The listing builds one solid part. Answer for the finished solid, in the listing's coordinates (mm). A direction names the side the tool comes from. Give positions to 0.01 mm unless a question says otherwise; leave off trailing zeros.
```python
from build123d import *

# Parameters (mm, degrees)
SKETCH1_W               = 60
SKETCH1_H               = 54.7
BOSS_EXTRUDE1_DEPTH     = 6.35
SKETCH2_W               = 15
SKETCH2_H               = 6
BOSS_EXTRUDE2_DEPTH     = 6.35
SKETCH3_R               = 1
CUT_EXTRUDE1_DEPTH      = 7.35
MIRROR2_COPY_1_SKETCH_W = 15
MIRROR2_COPY_1_SKETCH_H = 6
MIRROR2_COPY_1_DEPTH    = 6.35
MIRROR2_COPY_2_SKETCH_R = 1
MIRROR2_COPY_2_DEPTH    = 7.35
FILLET1_R               = 1
FILLET2_R               = 2


with BuildPart() as part:
    # Sketch1 → Boss-Extrude1 (new body)
    with BuildSketch(Plane.XY):
        Rectangle(SKETCH1_W, SKETCH1_H)
    extrude(amount=BOSS_EXTRUDE1_DEPTH)

    # Sketch2 → Boss-Extrude2 (add)
    with BuildSketch(Plane.XY.offset(6.35)):
        with Locations((-17.5, 30.35)):
            Rectangle(SKETCH2_W, SKETCH2_H)
    boss_extrude2 = extrude(amount=-BOSS_EXTRUDE2_DEPTH)

    # Sketch3 → Cut-Extrude1 (cut, through all)
    with BuildSketch(Plane.XY.offset(6.35)):
        with Locations((-25, 27.35)):
            Circle(SKETCH3_R)
        with Locations((-10, 27.35)):
            Circle(SKETCH3_R)
    cut_extrude1 = extrude(amount=-CUT_EXTRUDE1_DEPTH, mode=Mode.SUBTRACT)

    # Mirror1: Boss-Extrude2, Cut-Extrude1 across plane
    add(boss_extrude2.mirror(Plane(origin=(0, 0, 0), x_dir=(0, 0, 1), z_dir=(1, 0, 0))))
    add(cut_extrude1.mirror(Plane(origin=(0, 0, 0), x_dir=(0, 0, 1), z_dir=(1, 0, 0))), mode=Mode.SUBTRACT)

    # Mirror2: Boss-Extrude2, Cut-Extrude1 across plane
    add(boss_extrude2.mirror(Plane.ZX))
    add(cut_extrude1.mirror(Plane.ZX), mode=Mode.SUBTRACT)

    # Mirror2 copy 1 sketch → Mirror2 copy 1 (add)
    with BuildSketch(Plane(origin=(0, 0, 6.35), x_dir=(-1, 0, 0), z_dir=(0, 0, 1))):
        with Locations((-17.5, 30.35)):
            Rectangle(MIRROR2_COPY_1_SKETCH_W, MIRROR2_COPY_1_SKETCH_H)
    extrude(amount=-MIRROR2_COPY_1_DEPTH)

    # Mirror2 copy 2 sketch → Mirror2 copy 2 (cut, through all)
    with BuildSketch(Plane(origin=(0, 0, 6.35), x_dir=(-1, 0, 0), z_dir=(0, 0, 1))):
        with Locations((-25, 27.35)):
            Circle(MIRROR2_COPY_2_SKETCH_R)
        with Locations((-10, 27.35)):
            Circle(MIRROR2_COPY_2_SKETCH_R)
    extrude(amount=-MIRROR2_COPY_2_DEPTH, mode=Mode.SUBTRACT)

    # Fillet1
    fillet1_edges = [part.edges().sort_by_distance(p)[0] for p in [
        (26, -27.35, 3.175),
        (9, -27.35, 3.175),
        (-10, -33.35, 3.175),
        (-25, -33.35, 3.175),
        (-25, -28.35, 3.175),
        (-10, -28.35, 3.175),
        (-26, -27.35, 3.175),
        (-9, -27.35, 3.175),
        (-25, 33.35, 3.175),
        (-10, 33.35, 3.175),
        (-10, 28.35, 3.175),
        (-25, 28.35, 3.175),
        (-26, 27.35, 3.175),
        (-9, 27.35, 3.175),
        (10, 33.35, 3.175),
        (25, 33.35, 3.175),
        (25, 28.35, 3.175),
        (10, 28.35, 3.175),
        (26, 27.35, 3.175),
        (9, 27.35, 3.175),
        (25, -33.35, 3.175),
        (10, -33.35, 3.175),
        (10, -28.35, 3.175),
        (25, -28.35, 3.175),
    ]]
    fillet(fillet1_edges, radius=FILLET1_R)

    # Fillet2
    fillet2_edges = [part.edges().sort_by_distance(p)[0] for p in [
        (-30, 27.35, 3.175),
        (30, 27.35, 3.175),
        (30, -27.35, 3.175),
        (-30, -27.35, 3.175),
    ]]
    fillet(fillet2_edges, radius=FILLET2_R)


solid = part.part
```
Item 1: Each of these flat-tipped pins is pushed along its axis until it touches: P1, Ø1.4, axis at x = 27, z = 1.5, coming from the +Y side; P2, Ø3.5, axis at y = 31, z = 3.5, coming from the +X side; P3, Ø1, axis at y = -30, z = 3, coming from the -X side; P4, Ø1.2, axis at x = 25, y = -27.35, coming from the +Z side. Where does it stop, or does it pass through?
Conclusion:
P1: stops at y = 27.35
P2: stops at x = 25
P3: stops at x = -25
P4: passes through
Item 2: Which of the six approach directions +Z, -Z, +X, -X, +Y, -Y give full straight-line access (tool end or side, diameter ignored) to faces 5 (the face through (-25, -31, 3)), 6 (the face through (25, -31, 3)), 7 (the face through (0, -27.35, 3)), 8 (the face through (-25, 31, 3))?
Conclusion:
face 5: +Z, -Z, -X, -Y
face 6: +Z, -Z, +X, -Y
face 7: +Z, -Z, -Y
face 8: +Z, -Z, -X, +Y
Item 3: Determine the mould class of faces 1 (the face through (29.43, 26.75, 3.22)), 2 (the face through (-18, -33.35, 3)), 3 (the face through (10, 31, 3)), 4 (the face through (-10, -31, 3)) for opening direction X: pulls with the +X half, pulls with the -X half, needs draft (parallel to the pull), parting line crosses it, or undercut.
Conclusion:
face 1: pulls with the +X half
face 2: needs draft
face 3: undercut
face 4: undercut
Item 4: Consider probe 1 along X at (y, z) = (-30, 2); probe 2 along Y at (x, z) = (1, 3.5); probe 3 along Y at (x, z) = (-9.5, 1.75). Determine where each line is inside the solid, lowest interval first.
Conclusion:
probe 1: x = -25 to -10, 10 to 25
probe 2: y = -27.35 to 27.35
probe 3: y = -26.48 to 26.48
